The listing builds one solid part. Answer for the finished solid, in the listing's coordinates (mm). A direction names the side the tool comes from. Give positions to 0.01 mm unless a question says otherwise; leave off trailing zeros. Loops run counter-clockwise (first coordinate to the right, second up) from the corner with the lowest first, then second, coordinate; pieces in that order, holes last. Notation, with made-up numbers: (4, 82.5) - (12, 82.5) arc R26 cw to (12, 120.5) - close; hole circle Ø8 at (46, 18). An arc over 180 degrees is marked (long way). Write each question's results on one line, items separated by ' | '.
from build123d import *

# Parameters (mm, degrees)
F1_DEPTH = 20
F3_DEPTH = 1
F5_DEPTH = 4
F6_R     = 3
F7_DEPTH = 4
F8_R     = 6.5
F8_R_2   = 3
F9_DEPTH = 7


with BuildPart() as f1:
    # F0 (on Top) → F1 (new body)
    with BuildSketch(Plane.XY):
        with BuildLine():
            ThreePointArc((-24.1867732449, -12), (-27, 0), (-24.1867732449, 12))
            Line((-24.1867732449, 12), (-69.1867732449, 12))
            ThreePointArc((-69.1867732449, 12), (-72.7223071508, 10.5355339059), (-74.1867732449, 7))
            Line((-74.1867732449, 7), (-74.1867732449, -7))
            ThreePointArc((-74.1867732449, -7), (-72.7223071508, -10.5355339059), (-69.1867732449, -12))
            Line((-69.1867732449, -12), (-24.1867732449, -12))
        make_face()
        with BuildLine():
            ThreePointArc((24.1867732449, -12), (26.2872866383, -6.1626748408), (27, 0))
            ThreePointArc((27, 0), (26.2872866383, 6.1626748408), (24.1867732449, 12))
            ThreePointArc((24.1867732449, 12), (19.091883092, 19.091883092), (12, 24.1867732449))
            ThreePointArc((12, 24.1867732449), (0, 27), (-12, 24.1867732449))
            ThreePointArc((-12, 24.1867732449), (-19.091883092, 19.091883092), (-24.1867732449, 12))
            ThreePointArc((-24.1867732449, 12), (-27, 0), (-24.1867732449, -12))
            ThreePointArc((-24.1867732449, -12), (-19.091883092, -19.091883092), (-12, -24.1867732449))
            ThreePointArc((-12, -24.1867732449), (0, -27), (12, -24.1867732449))
            ThreePointArc((12, -24.1867732449), (19.091883092, -19.091883092), (24.1867732449, -12))
        make_face()
        with BuildLine():
            ThreePointArc((3, 23.1060598112), (17.5041423669, 15.3783939343), (23.3, 0))
            ThreePointArc((23.3, 0), (17.5041423669, -15.3783939343), (3, -23.1060598112))
            ThreePointArc((3, -23.1060598112), (0, -23.3), (-3, -23.1060598112))
            ThreePointArc((-3, -23.1060598112), (-16.4755880016, -16.4755880016), (-23.1060598112, -3))
            ThreePointArc((-23.1060598112, -3), (-23.3, 0), (-23.1060598112, 3))
            ThreePointArc((-23.1060598112, 3), (-16.4755880016, 16.4755880016), (-3, 23.1060598112))
            ThreePointArc((-3, 23.1060598112), (0, 23.3), (3, 23.1060598112))
        make_face(mode=Mode.SUBTRACT)
        with BuildLine():
            Line((-3, 7.9529868603), (-3, 23.1060598112))
            ThreePointArc((-3, 23.1060598112), (-16.4755880016, 16.4755880016), (-23.1060598112, 3))
            Line((-23.1060598112, 3), (-7.9529868603, 3))
            ThreePointArc((-7.9529868603, 3), (-6.0104076401, 6.0104076401), (-3, 7.9529868603))
        make_face()
        with BuildLine():
            ThreePointArc((3, -23.1060598112), (17.5041423669, -15.3783939343), (23.3, 0))
            ThreePointArc((23.3, 0), (17.5041423669, 15.3783939343), (3, 23.1060598112))
            Line((3, 23.1060598112), (3, 7.9529868603))
            ThreePointArc((3, 7.9529868603), (6.0104076401, 6.0104076401), (7.9529868603, 3))
            Line((7.9529868603, 3), (17.3, 3))
            Line((17.3, 3), (17.3, -3))
            Line((17.3, -3), (7.9529868603, -3))
            ThreePointArc((7.9529868603, -3), (6.0104076401, -6.0104076401), (3, -7.9529868603))
            Line((3, -7.9529868603), (3, -23.1060598112))
        make_face()
        with BuildLine():
            ThreePointArc((-23.1060598112, -3), (-16.4755880016, -16.4755880016), (-3, -23.1060598112))
            Line((-3, -23.1060598112), (-3, -7.9529868603))
            ThreePointArc((-3, -7.9529868603), (-6.0104076401, -6.0104076401), (-7.9529868603, -3))
            Line((-7.9529868603, -3), (-23.1060598112, -3))
        make_face()
        with BuildLine():
            ThreePointArc((-12, 24.1867732449), (0, 27), (12, 24.1867732449))
            Line((12, 24.1867732449), (12, 69.1867732449))
            ThreePointArc((12, 69.1867732449), (10.5355339059, 72.7223071508), (7, 74.1867732449))
            Line((7, 74.1867732449), (-7, 74.1867732449))
            ThreePointArc((-7, 74.1867732449), (-10.5355339059, 72.7223071508), (-12, 69.1867732449))
            Line((-12, 69.1867732449), (-12, 24.1867732449))
        make_face()
        with BuildLine():
            ThreePointArc((24.1867732449, 12), (26.2872866383, 6.1626748408), (27, 0))
            ThreePointArc((27, 0), (26.2872866383, -6.1626748408), (24.1867732449, -12))
            Line((24.1867732449, -12), (69.1867732449, -12))
            ThreePointArc((69.1867732449, -12), (72.7223071508, -10.5355339059), (74.1867732449, -7))
            Line((74.1867732449, -7), (74.1867732449, 7))
            ThreePointArc((74.1867732449, 7), (72.7223071508, 10.5355339059), (69.1867732449, 12))
            Line((69.1867732449, 12), (24.1867732449, 12))
        make_face()
        with BuildLine():
            Line((12, -69.1867732449), (12, -24.1867732449))
            ThreePointArc((12, -24.1867732449), (0, -27), (-12, -24.1867732449))
            Line((-12, -24.1867732449), (-12, -69.1867732449))
            ThreePointArc((-12, -69.1867732449), (-10.5355339059, -72.7223071508), (-7, -74.1867732449))
            Line((-7, -74.1867732449), (7, -74.1867732449))
            ThreePointArc((7, -74.1867732449), (10.5355339059, -72.7223071508), (12, -69.1867732449))
        make_face()
    extrude(amount=F1_DEPTH)

    # F2 (on face) → F3 (cut)
    with BuildSketch(Plane.XY.offset(20)):
        with BuildLine():
            Line((3, -74.1867732449), (3, -23.1060598112))
            ThreePointArc((3, -23.1060598112), (0, -23.3), (-3, -23.1060598112))
            Line((-3, -23.1060598112), (-3, -7.9529868603))
            ThreePointArc((-3, -7.9529868603), (-6.0104076401, -6.0104076401), (-7.9529868603, -3))
            Line((-7.9529868603, -3), (-23.1060598112, -3))
            ThreePointArc((-23.1060598112, -3), (-23.3, 0), (-23.1060598112, 3))
            Line((-23.1060598112, 3), (-74.1867732449, 3))
            Line((-74.1867732449, 3), (-74.1867732449, -7))
            ThreePointArc((-74.1867732449, -7), (-72.7223071508, -10.5355339059), (-69.1867732449, -12))
            Line((-69.1867732449, -12), (-24.1867732449, -12))
            ThreePointArc((-24.1867732449, -12), (-19.091883092, -19.091883092), (-12, -24.1867732449))
            Line((-12, -24.1867732449), (-12, -69.1867732449))
            ThreePointArc((-12, -69.1867732449), (-10.5355339059, -72.7223071508), (-7, -74.1867732449))
            Line((-7, -74.1867732449), (3, -74.1867732449))
        make_face()
    extrude(amount=-F3_DEPTH, mode=Mode.SUBTRACT)

    # F4 (on face) → F5 (cut)
    with BuildSketch(Plane.XY.offset(19)):
        with BuildLine():
            ThreePointArc((-8.6168439698, -4), (-6.7175144213, -6.7175144213), (-4, -8.6168439698))
            Line((-4, -8.6168439698), (-4, -23.1060598112))
            Line((-4, -23.1060598112), (-3, -23.1060598112))
            Line((-3, -23.1060598112), (-3, -7.9529868603))
            ThreePointArc((-3, -7.9529868603), (-6.0104076401, -6.0104076401), (-7.9529868603, -3))
            Line((-7.9529868603, -3), (-23.1060598112, -3))
            Line((-23.1060598112, -3), (-23.1060598112, -4))
            Line((-23.1060598112, -4), (-8.6168439698, -4))
        make_face()
    extrude(amount=-F5_DEPTH, mode=Mode.SUBTRACT)

    # F6 (on face) → F7 (join)
    with BuildSketch(Plane(origin=(0, 0, 0), x_dir=(1, 0, 0), z_dir=(0, 0, -1))):
        with BuildLine():
            ThreePointArc((-74.1867732449, -7), (-72.7223071508, -10.5355339059), (-69.1867732449, -12))
            Line((-69.1867732449, -12), (-24.1867732449, -12))
            ThreePointArc((-24.1867732449, -12), (-19.091883092, -19.091883092), (-12, -24.1867732449))
            Line((-12, -24.1867732449), (-12, -69.1867732449))
            ThreePointArc((-12, -69.1867732449), (-10.5355339059, -72.7223071508), (-7, -74.1867732449))
            Line((-7, -74.1867732449), (7, -74.1867732449))
            ThreePointArc((7, -74.1867732449), (10.5355339059, -72.7223071508), (12, -69.1867732449))
            Line((12, -69.1867732449), (12, -24.1867732449))
            ThreePointArc((12, -24.1867732449), (19.091883092, -19.091883092), (24.1867732449, -12))
            Line((24.1867732449, -12), (69.1867732449, -12))
            ThreePointArc((69.1867732449, -12), (72.7223071508, -10.5355339059), (74.1867732449, -7))
            Line((74.1867732449, -7), (74.1867732449, 7))
            ThreePointArc((74.1867732449, 7), (72.7223071508, 10.5355339059), (69.1867732449, 12))
            Line((69.1867732449, 12), (24.1867732449, 12))
            ThreePointArc((24.1867732449, 12), (19.091883092, 19.091883092), (12, 24.1867732449))
            Line((12, 24.1867732449), (12, 69.1867732449))
            ThreePointArc((12, 69.1867732449), (10.5355339059, 72.7223071508), (7, 74.1867732449))
            Line((7, 74.1867732449), (-7, 74.1867732449))
            ThreePointArc((-7, 74.1867732449), (-10.5355339059, 72.7223071508), (-12, 69.1867732449))
            Line((-12, 69.1867732449), (-12, 24.1867732449))
            ThreePointArc((-12, 24.1867732449), (-19.091883092, 19.091883092), (-24.1867732449, 12))
            Line((-24.1867732449, 12), (-69.1867732449, 12))
            ThreePointArc((-69.1867732449, 12), (-72.7223071508, 10.5355339059), (-74.1867732449, 7))
            Line((-74.1867732449, 7), (-74.1867732449, -7))
        make_face()
        with BuildLine():
            Line((3, -7.9529868603), (3, -23.1060598112))
            ThreePointArc((3, -23.1060598112), (0, -23.3), (-3, -23.1060598112))
            Line((-3, -23.1060598112), (-3, -7.9529868603))
            ThreePointArc((-3, -7.9529868603), (-6.0104076401, -6.0104076401), (-7.9529868603, -3))
            Line((-7.9529868603, -3), (-23.1060598112, -3))
            ThreePointArc((-23.1060598112, -3), (-23.3, 0), (-23.1060598112, 3))
            Line((-23.1060598112, 3), (-7.9529868603, 3))
            ThreePointArc((-7.9529868603, 3), (-6.0104076401, 6.0104076401), (-3, 7.9529868603))
            Line((-3, 7.9529868603), (-3, 23.1060598112))
            ThreePointArc((-3, 23.1060598112), (0, 23.3), (3, 23.1060598112))
            Line((3, 23.1060598112), (3, 7.9529868603))
            ThreePointArc((3, 7.9529868603), (6.0104076401, 6.0104076401), (7.9529868603, 3))
            Line((7.9529868603, 3), (17.3, 3))
            Line((17.3, 3), (17.3, -3))
            Line((17.3, -3), (7.9529868603, -3))
            ThreePointArc((7.9529868603, -3), (6.0104076401, -6.0104076401), (3, -7.9529868603))
        make_face(mode=Mode.SUBTRACT)
        with BuildLine():
            ThreePointArc((-3, -23.1060598112), (0, -23.3), (3, -23.1060598112))
            Line((3, -23.1060598112), (3, -7.9529868603))
            ThreePointArc((3, -7.9529868603), (6.0104076401, -6.0104076401), (7.9529868603, -3))
            Line((7.9529868603, -3), (17.3, -3))
            Line((17.3, -3), (17.3, 3))
            Line((17.3, 3), (7.9529868603, 3))
            ThreePointArc((7.9529868603, 3), (6.0104076401, 6.0104076401), (3, 7.9529868603))
            Line((3, 7.9529868603), (3, 23.1060598112))
            ThreePointArc((3, 23.1060598112), (0, 23.3), (-3, 23.1060598112))
            Line((-3, 23.1060598112), (-3, 7.9529868603))
            ThreePointArc((-3, 7.9529868603), (-6.0104076401, 6.0104076401), (-7.9529868603, 3))
            Line((-7.9529868603, 3), (-23.1060598112, 3))
            ThreePointArc((-23.1060598112, 3), (-23.3, 0), (-23.1060598112, -3))
            Line((-23.1060598112, -3), (-7.9529868603, -3))
            ThreePointArc((-7.9529868603, -3), (-6.0104076401, -6.0104076401), (-3, -7.9529868603))
            Line((-3, -7.9529868603), (-3, -23.1060598112))
        make_face()
        Circle(F6_R, mode=Mode.SUBTRACT)
    extrude(amount=-F7_DEPTH)

    # F8 (on face) → F9 (join)
    with BuildSketch(Plane.XY.offset(4)):
        Circle(F8_R)
        Circle(F8_R_2, mode=Mode.SUBTRACT)
    extrude(amount=F9_DEPTH)


solid = f1.part
Item 1: For faces 4 (the face through (19.179, 19.005, 9.86)), 5 (the face through (12, -47, 10)), 6 (the face through (-12, 47, 10)), 7 (the face through (-6.05, 5.97, 11.89)), 8 (the face through (-72.76, -10.5, 9.37)), determine the directions among +Z, -Z, +X, -X, +Y, -Y from which every point of the face is accessible in a straight line to the end or side of a thin tool.
Values found:
face 4: +Z, -Z, +X, +Y | face 5: +Z, -Z, +X, -Y | face 6: +Z, -Z, -X, +Y | face 7: +Z | face 8: +Z, -Z, -X, -Y
Item 2: A cutting plane is placed at D-D, the plane y = -35.5. Determine the outline of the cut face in (x, z), plus the area to 3 significant figures.
Values found:
outline: (-12, 0) - (12, 0) - (12, 20) - (3, 20) - (3, 19) - (-12, 19) - close | area: 465 mm²
Item 3: Find the intervals of material crossed by line 1 along Y through (x, z) = (0, 8.75); line 2 along X through (y, z) = (-2, 6); line 3 along X through (y, z) = (0, 0.8), in increasing order. Write a range as [from, to].
Values found:
line 1: y = [-74.19, -23.3], [-6.5, -3], [3, 6.5], [23.3, 74.19] | line 2: x = [-74.19, -23.21], [-6.18, -2.24], [2.24, 6.18], [17.3, 74.19] | line 3: x = [-74.19, -3], [3, 74.19]
Item 4: A cutting plane is placed at C-C, the plane z = 9.25. Count the separate pieces of the cut face and the enclosed holes in it, plus the area to 3 significant figures.
Values found:
separate pieces: 2 | enclosed holes: 2 | area: 6,420 mm²
Item 5: Flat-ended cylindrical pins translate along their axes: P1, Ø10, axis at x = 9.5, z = 12.5, coming from the +Y side; P2, Ø5, axis at x = -36, z = 11, coming from the -Y side; P3, Ø1, axis at y = -13, z = 4, coming from the -X side; P4, Ø6.5, axis at x = -2, y = 1.5, coming from the +Z side. Find the tip coordinate at first contact, or state that the pin passes through.
Values found:
P1: stops at y = 74.19 | P2: stops at y = -12 | P3: stops at x = -23.93 | P4: stops at z = 11
Item 6: A cutting plane is placed at A-A, the plane y = 0. Determine the outline of the cut face in (x, z).
Values found:
outline: (-74.19, 0) - (-3, 0) - (-3, 11) - (-6.5, 11) - (-6.5, 4) - (-23.3, 4) - (-23.3, 19) - (-74.19, 19) - close; (3, 0) - (74.19, 0) - (74.19, 20) - (17.3, 20) - (17.3, 4) - (6.5, 4) - (6.5, 11) - (3, 11) - close
Item 7: A cutting plane is placed at B-B, the plane x = 0. Determine the outline of the cut face in (y, z), plus the area to 3 significant figures.
Values found:
outline: (-74.19, 0) - (-3, 0) - (-3, 11) - (-6.5, 11) - (-6.5, 4) - (-23.3, 4) - (-23.3, 19) - (-74.19, 19) - close; (3, 0) - (74.19, 0) - (74.19, 20) - (23.3, 20) - (23.3, 4) - (6.5, 4) - (6.5, 11) - (3, 11) - close | area: 2,200 mm²
Item 8: For a pull along X with two mould halves and no side action, classify faces 1 (the face through (-10.574, -72.683, 9.367)), 2 (the face through (3, 16, 12)), 3 (the face through (12, 46, 10)) as released by +X, released by -X, zero draft, split by the parting line, or undercut.
Values found:
face 1: released by -X | face 2: undercut | face 3: released by +X
